Geometry check sheet. Reference: the model listing, model coordinates, mm. A direction names the side the tool comes from. Round coordinates to 2 decimals unless told otherwise and drop trailing zeros. Loops run counter-clockwise (first coordinate to the right, second up) from the corner with the lowest first, then second, coordinate; pieces in that order, holes last.
```python
from build123d import *

# Parameters (mm, degrees)
F0_W     = 61.6968180984
F0_H     = 68.7478855252
F1_DEPTH = 50.8
F2_DEPTH = 25.4
F3_DEPTH = 25.4
F5_W     = 33.1008322537
F5_H     = 32.9049695283
F6_DEPTH = 114.40052
F7_DEPTH = 76.93265
F8_DEPTH = 127
F9_DEPTH = 80.68794


with BuildPart() as f1:
    # F0 (on Front) → F1 (new body)
    with BuildSketch(Plane.XZ):
        with Locations((-2.2524232045, 0.7834509015)):
            Rectangle(F0_W, F0_H)
    extrude(amount=F1_DEPTH)

    # F2 (add): faces of the model
    f2_faces = [f1.faces().sort_by_distance(p)[0] for p in [
        (-2.2524232045, -50.8, 0.7834509015),
        (-2.2524232045, 0, 0.7834509015),
    ]]
    extrude(f2_faces, amount=F2_DEPTH, dir=(0, -1, 0))

    # F3 (add): a face of the model
    f3_faces = [f1.faces().sort_by_distance(p)[0] for p in [
        (-2.2524232045, -76.2, 0.7834509015),
    ]]
    extrude(f3_faces, amount=F3_DEPTH)

    # F5 (on face) → F6 (join)
    with BuildSketch(Plane.XZ.offset(101.6)):
        with Locations((-16.5504161268, 4.0151895955)):
            Rectangle(F5_W, F5_H)
    extrude(amount=-F6_DEPTH)

    # F7 (add): a face of the model
    f7_faces = [f1.faces().sort_by_distance(p)[0] for p in [
        (-16.5504161268, 12.80052, 4.0151895955),
    ]]
    extrude(f7_faces, amount=-F7_DEPTH)

    # F8 (add): a face of the model
    f8_faces = [f1.faces().sort_by_distance(p)[0] for p in [
        (-16.5504161268, 12.80052, 4.0151895955),
    ]]
    extrude(f8_faces, amount=-F8_DEPTH)

    # F9 (add): a face of the model
    f9_faces = [f1.faces().sort_by_distance(p)[0] for p in [
        (-16.5504161268, -114.19948, 4.0151895955),
    ]]
    extrude(f9_faces, amount=-F9_DEPTH)


solid = f1.part
```
1) Sectioned sample at B-B, the plane x = -22. Record the cut outline in (y, z).
Report:
outline: (-114.2, -12.44) - (-101.6, -12.44) - (-101.6, -33.59) - (0, -33.59) - (0, -12.44) - (12.8, -12.44) - (12.8, 20.47) - (0, 20.47) - (0, 35.16) - (-101.6, 35.16) - (-101.6, 20.47) - (-114.2, 20.47) - close
2) Sectioned sample at D-D, the plane x = 19.5. Record the cut outline in (y, z), then the cut area to 3 significant figures.
Report:
outline: (-101.6, -33.59) - (0, -33.59) - (0, 35.16) - (-101.6, 35.16) - close
area: 6,980 mm2
3) Gauge pin test, flat ends, axial feed: pin 1 (4 mm diameter, centred on x = -13.5, y = -110.5, fed in from +Z); pin 2 (4 mm diameter, centred on y = 5.5, z = -0.5, fed in from +X); pin 3 (10 mm diameter, centred on x = -13.5, y = 7.5, fed in from -Z). Record the tip position at first contact, or that the pin passes through.
Report:
pin 1: stops at z = 20.47
pin 2: stops at x = 0
pin 3: stops at z = -12.44
4) Access from +Z, -Z, +X, -X, +Y, -Y to the whole of each face (thin tool, end or side, straight path). Record for faces 1 (the face through (-17, -108, -12.437)), 2 (the face through (-17, 6, 20.468)), 3 (the face through (0, 6, 4)), 4 (the face through (-17, 6, -12.437)), 5 (the face through (-17, -108, 20.468)).
Report:
face 1: -Z, +X, -X, -Y
face 2: +Z, +X, -X, +Y
face 3: +Z, -Z, +X, +Y
face 4: -Z, +X, -X, +Y
face 5: +Z, +X, -X, -Y
5) Sectioned sample at A-A, the plane z = 18.5. Record the cut outline in (x, y), then the cut area to 3 significant figures.
Report:
outline: (-33.1, -114.2) - (0, -114.2) - (0, -101.6) - (28.6, -101.6) - (28.6, 0) - (0, 0) - (0, 12.8) - (-33.1, 12.8) - close
area: 7,110 mm2
6) Scan lines: line 1 along Z through (x, y) = (-3.5, -103.5); line 2 along Y through (x, z) = (15, 3.5); line 3 along X through (y, z) = (3, 17). Record each from-to range of solid material in increasing order.
Report:
line 1: z = -12.44 to 20.47
line 2: y = -101.6 to 0
line 3: x = -33.1 to 0
7) Sectioned sample at C-C, the plane y = 5.5. Record the cut outline in (x, z), then the cut area to 3 significant figures.
Report:
outline: (-33.1, -12.44) - (0, -12.44) - (0, 20.47) - (-33.1, 20.47) - close
area: 1,090 mm2
